For this review, use the dimensioned drawing (mm, ordinates from the lowest corner) and the shaded views. Give positions to 0.01 mm unless a question says otherwise; leave off trailing zeros. Order: outer loops, then holes, each group sorted by start corner. A loop starts at its lowest first (then second) coordinate and runs counter-clockwise, first axis right, second up. Notation, with made-up numbers: (86.5, 19.5) -> (132.5, 19.5) arc R10 cw to (132.5, 34.5) -> close; hole circle Ø1 at (44.25, -9). An arc over 180 degrees is marked (long way). One line per item, written item: value. Start each with the question number.
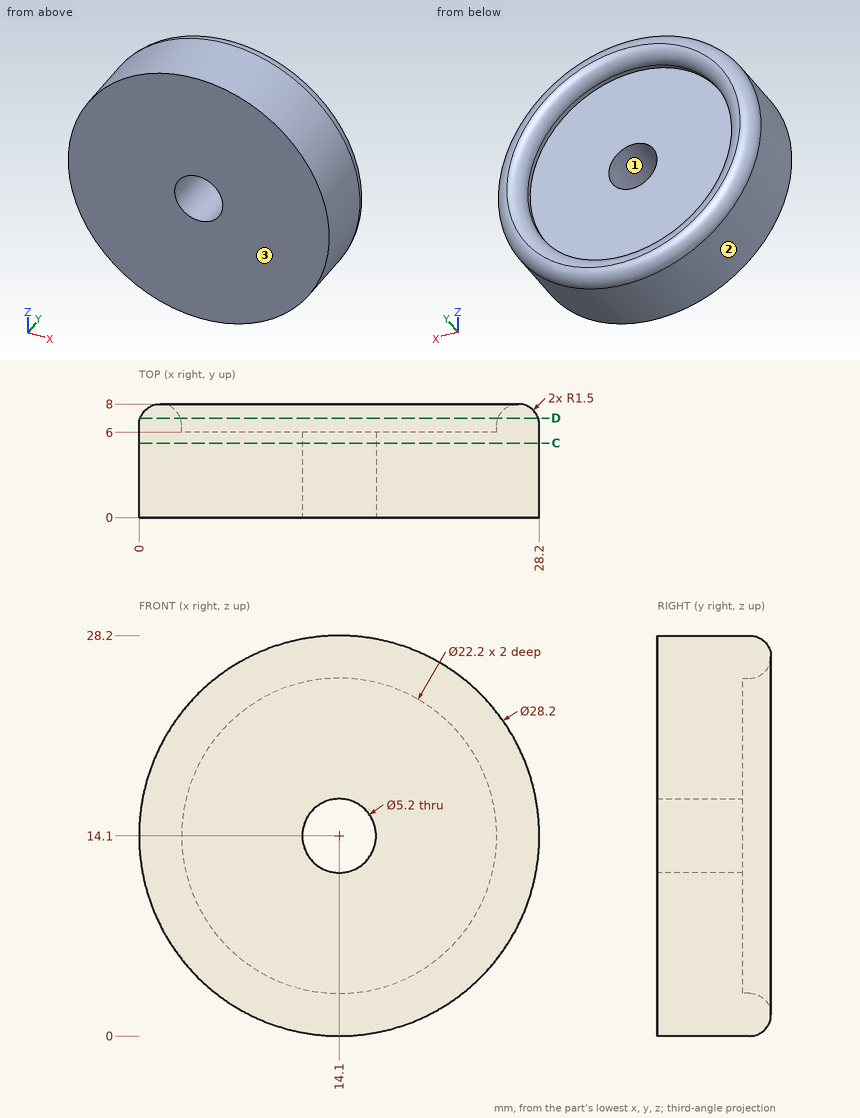
Q1. For line 1 along X through (y, z) = (6.4, 14.1); line 2 along X through (y, z) = (1.55, 14.1); line 3 along Y through (x, z) = (14.75, 11), list the stretches that pass through material, from the lowest coordinate up.
Q2. For pin 1 Ø4 at (y, z) = (2.5, 3.5) entering from -X; pin 2 Ø4 at (y, z) = (3, 11) entering from -X; pin 3 Ø3 at (y, z) = (1.5, 23) entering from +X, all flat-tipped, find the tip position at first contact; note any pin that passes through.
Q3. Mouldability with a two-part tool opening along Z and no side actions: class the marked faces 1, 2 and 3 as pulls with the +Z half, pulls with the -Z half, needs draft (parallel to the pull), parting line crosses it, or undercut.
Q4. Take a section at D-D (y = 7). State the section outline as (x, z) points.
Q5. Take a section at C-C (y = 5.25). State the section outline as (x, z) points, and give its area (3 significant figures).
Answers below:
1. line 1: x = 0 to 3, 25.2 to 28.2
1. line 2: x = 0 to 11.5, 16.7 to 28.2
1. line 3: y = 0 to 6
2. pin 1: stops at x = 2.93
2. pin 2: stops at x = 0.04
2. pin 3: stops at x = 26.1
3. face 1: undercut
3. face 2: parting line crosses it
3. face 3: needs draft
4. outline: circle Ø28.03 at (14.1, 14.1); hole circle Ø22.37 at (14.1, 14.1)
5. outline: circle Ø28.2 at (14.1, 14.1); hole circle Ø5.2 at (14.1, 14.1)
5. area: 603 mm²
